Here's how the part is built. I have some questions about the finished solid (model axes, mm). Face numbers are marked on the shaded views. A direction names the side the tool comes from. Give positions to 0.01 mm unless a question says otherwise; leave off trailing zeros. Loops run counter-clockwise (first coordinate to the right, second up) from the corner with the lowest first, then second, coordinate; pieces in that order, holes last. Notation, with made-up numbers: M 70.25,50.25 L 80.25,50.25 A21 cw 80.25,86.25 Z; hole C 45,47.25 d4. An arc over 180 degrees is marked long. Answer as CSV lines item,"result". Start each with the question number.
Item 1: I want a section at A-A on x = -15.5. List the corners of the cut face in (y, z) for me.
Item 2: If I drill on line 1 along X through (y, z) = (-2.5, 1); line 2 along Y through (x, z) = (-15.5, -3.25); line 3 along Y through (x, z) = (-6.5, 0.75), over which ranges is the centre line in solid material (lowest first)? Write a range as from..to.
Item 3: I want a section at C-C on y = 4.75. List the corners of the cut face in (x, z) for me, plus the area to 3 significant figures.
Item 4: If we mould it in two halves opening along Y, with no side actions, what happens to the marked faces 3, 4 and 5? For each: released by +Y, released by -Y, zero draft, split by the parting line, or undercut.
Item 5: I want a section at B-B on x = 10. List the corners of the cut face in (y, z) for me, plus the area to 3 significant figures.
Item 6: I want a section at D-D on z = -4. Give the number of separate pieces and of enclosed holes in the cut face, plus the area to 3 significant figures.
Item 7: For the marked faces 1 and 2, which set-ups out of +Z, -Z, +X, -X, +Y, -Y let a thin tool reach every point of the face, with its end or its side?
Item 8: Will these pins go through, and if not, where does the flat tip stop? P1, Ø0.6, axis at x = 4.5, y = -4.5, coming from the -Z side; P2, Ø1, axis at x = 6, z = -5, coming from the +Y side; P3, Ø5, axis at x = 5, y = 9.5, coming from the +Z side.
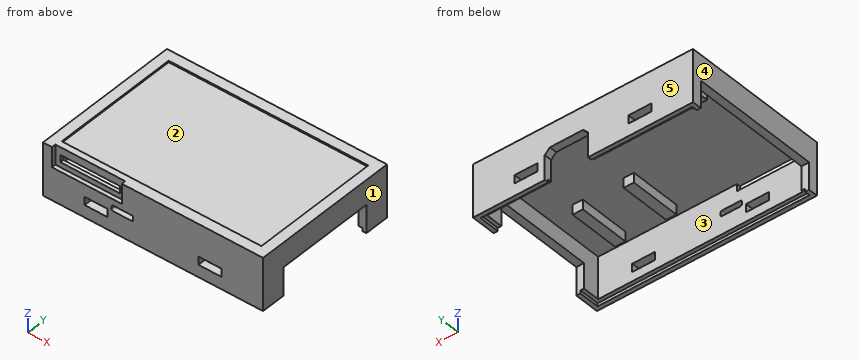
Autodesk Inventor part; units mm, degrees
ref_plane "EbeneAuflage" through (-20, -13, 0) normal (0, 0, 1) x (1, 0, 0)
ref_plane "YZ Plane" through (0, 0, 0) normal (1, 0, 0) x (0, 1, 0)
ref_plane "XZ Plane" through (0, 0, 0) normal (0, 1, 0) x (-1, 0, 0)
ref_plane "EbeneBoden" through (-11.5031, -4.6031, 1.9) normal (0, 0, 1) x (1, 0, 0)
ref_plane "EbeneWändeEnde" through (17.7, 4.9, -6.9) normal (0, 0, -1) x (-1, 0, 0)
sketch "SkizzeBoden" plane through (-11.5031, -4.6031, 1.9) normal (0, 0, 1) x (1, 0, 0)
  line L0 (-7.1969, 7.4031) -> (6.8031, 7.4031)
  line L1 (6.8031, 7.4031) -> (6.8031, -7.7969)
  line L2 (6.8031, -7.7969) -> (4.3031, -7.7969)
  line L3 (4.3031, -7.7969) -> (4.3031, -6.7969)
  line L4 (4.3031, -6.7969) -> (-7.1969, -6.7969)
  line L5 (-7.1969, -6.7969) -> (-7.1969, 7.4031)
  line L6 (31.5031, 17.6031) -> (-8.4969, 17.6031)
  line L7 (-8.4969, 17.6031) -> (-8.4969, -8.3969)
  line L8 (-8.4969, -8.3969) -> (31.5031, -8.3969)
  line L9 (31.5031, -8.3969) -> (31.5031, 17.6031)
  line L10 (-18.6669, 4.6031) -> (41.6731, 4.6031)
  line L11 (11.5031, -15.7669) -> (11.5031, 24.9731)
  line L12 (-10.0469, 19.1531) -> (33.0531, 19.1531)
  line L13 (33.0531, 19.1531) -> (33.0531, -9.9469)
  line L14 (33.0531, -9.9469) -> (-10.0469, -9.9469)
  line L15 (-10.0469, -9.9469) -> (-10.0469, 19.1531)
  point P0 (11.5031, 4.6031)
  dimension "d0" = 1.55
extrude "Boden" add sketch "SkizzeBoden" along normal blind 1.5
sketch "SkizzeWände" plane through (-11.5031, -4.6031, 1.9) normal (0, 0, -1) x (-1, 0, 0)
  line L0 (10.0469, 19.1531) -> (-33.0531, 19.1531)
  line L1 (-33.0531, 19.1531) -> (-33.0531, -9.9469)
  line L2 (-33.0531, -9.9469) -> (10.0469, -9.9469)
  line L3 (10.0469, -9.9469) -> (10.0469, 19.1531)
  line L4 (-31.5531, 17.6531) -> (8.5469, 17.6531)
  line L5 (8.5469, 17.6531) -> (8.5469, -8.4469)
  line L6 (8.5469, -8.4469) -> (-31.5531, -8.4469)
  line L7 (-31.5531, -8.4469) -> (-31.5531, 17.6531)
  point P0 (-11.5031, 4.6031)
  dimension "d3" = 1.5
extrude "Wände" add sketch "SkizzeWände" along normal up to surface (8.8 mm away)
sketch "SkizzeAuflage" plane through (-11.5031, -4.6031, 1.9) normal (0, 0, -1) x (-1, 0, 0)
  line L0 (8.5469, -8.4469) -> (8.5469, 17.6531)
  line L1 (-31.5531, -8.4469) -> (8.5469, -8.4469)
  line L2 (-31.5531, 17.6531) -> (-31.5531, -8.4469)
  line L3 (8.5469, 17.6531) -> (-31.5531, 17.6531)
  line L4 (10.0469, 19.1531) -> (10.0469, -9.9469)
  line L5 (-33.0531, 19.1531) -> (10.0469, 19.1531)
  line L6 (-33.0531, -9.9469) -> (-33.0531, 19.1531)
  line L7 (10.0469, -9.9469) -> (-33.0531, -9.9469)
  line L8 (-26.5531, 3.5531) -> (-24.5531, 3.5531)
  line L9 (-24.5531, 3.5531) -> (-24.5531, -6.4469)
  line L10 (-24.5531, -6.4469) -> (-26.5531, -6.4469)
  line L11 (-26.5531, -6.4469) -> (-26.5531, 3.5531)
  line L12 (-16.5531, 3.5531) -> (-14.5531, 3.5531)
  line L13 (-14.5531, 3.5531) -> (-14.5531, -6.4469)
  line L14 (-14.5531, -6.4469) -> (-16.5531, -6.4469)
  line L15 (-16.5531, -6.4469) -> (-16.5531, 3.5531)
  line L16 (6.5469, 13.6531) -> (-13.4531, 13.6531)
  line L17 (-13.4531, 13.6531) -> (-13.4531, 11.6531)
  line L18 (-13.4531, 11.6531) -> (6.5469, 11.6531)
  line L19 (6.5469, 11.6531) -> (6.5469, 13.6531)
  point P0 (-11.5031, 4.6031)
  dimension "d6" = 5
  dimension "d7" = 2
  dimension "d8" = 8
  dimension "d9" = 2
  dimension "d10" = 10
  dimension "d11" = 20
  dimension "d12" = 2
  dimension "d13" = 4
  dimension "d14" = 2
ref_plane "EbeneAuflage" through (-20, -13, 0) normal (0, 0, 1) x (1, 0, 0)
extrude "Auflage" add sketch "SkizzeAuflage" along normal up to surface (1.9 mm away) contours L8 L9 L10 L11 | L12 L13 L14 L15 | L19 L18 L17 L16
sketch "SkizzeSD" plane through (-21.55, -14.55, 3.4) normal (0, -1, 0) x (1, 0, 0)
  line L0 (43.1, 0) -> (43.1, -10.3)
  line L1 (3.05, -2.6) -> (14.15, -2.6)
  line L2 (14.15, -2.6) -> (14.15, -1.6)
  line L3 (14.15, -1.6) -> (3.05, -1.6)
  line L4 (3.05, -1.6) -> (3.05, -2.6)
  line L5 (41.6, -1.5) -> (1.5, -1.5)
  line L6 (14.45, -1.5) -> (2.75, -1.5)
  line L7 (2.75, -1.5) -> (2.75, -2.9)
  line L8 (2.75, -2.9) -> (14.45, -2.9)
  line L9 (14.45, -2.9) -> (14.45, -1.5)
  line L10 (8.6, -4) -> (8.6, -0.8838) construction
  point P0 (21.55, -3.4)
  point P1 (8.6, -2.6)
  dimension "d17" = 0.3
  dimension "d18" = 0.3
extrude "SD" cut sketch "SkizzeSD" against normal up to surface (1.5 mm away) contours L4 L3 L2 L1 | L9 L8 L7 L5
sketch "Skizze7" plane through (-21.55, -14.55, 3.4) normal (0, -1, 0) x (1, 0, 0)
  line L0 (14.45, -1.5) -> (14.45, -2.9)
  line L1 (14.45, -2.9) -> (2.75, -2.9)
  line L2 (0, 0) -> (43.1, 0)
  line L3 (15.45, -3.9) -> (1.75, -3.9)
  line L4 (1.75, -3.9) -> (1.75, 0)
  line L5 (1.75, 0) -> (15.45, 0)
  line L6 (15.45, 0) -> (15.45, -3.9)
  line L7 (8.6, -3.6567) -> (8.6, -1) construction
  point P0 (21.55, -3.4)
  point P1 (8.6, -2.9)
  dimension "d21" = 1
  dimension "d22" = 1
extrude "SDHilfe" cut sketch "Skizze7" against normal blind 0.8
sketch "SkizzeLED" plane through (-21.55, -14.55, -6.9) normal (0, -1, 0) x (1, 0, 0)
  line L0 (16.55, 5.2) -> (17.55, 5.2)
  line L1 (16.55, 5.2) -> (16.55, 4.1)
  line L2 (17.55, 4.1) -> (16.55, 4.1)
  line L3 (17.55, 5.2) -> (17.55, 4.1)
  line L4 (15.05, 5.2) -> (16.05, 5.2)
  line L5 (15.05, 5.2) -> (15.05, 4.1)
  line L6 (16.05, 4.1) -> (15.05, 4.1)
  line L7 (16.05, 5.2) -> (16.05, 4.1)
  line L8 (13.55, 5.2) -> (14.55, 5.2)
  line L9 (13.55, 5.2) -> (13.55, 4.1)
  line L10 (14.55, 4.1) -> (13.55, 4.1)
  line L11 (14.55, 5.2) -> (14.55, 4.1)
  line L12 (15.55, 3.5363) -> (15.55, 5.4531) construction
  line L13 (17.65, 4.1) -> (13.45, 4.1)
  line L14 (13.45, 4.1) -> (13.45, 5.2)
  line L15 (13.45, 5.2) -> (17.65, 5.2)
  line L16 (17.65, 5.2) -> (17.65, 4.1)
  line L17 (41.55, 5.2) -> (1.55, 5.2)
  point P0 (21.55, 6.9)
  point P1 (15.55, 4.1)
  dimension "d25" = 0.1
extrude "LED" cut sketch "SkizzeLED" against normal up to surface (1.5 mm away)
fillet "RundungLED" radius 0.3 4 edges at (-8.1, -13.8, -2.8) (-3.9, -13.8, -2.8) (-8.1, -13.8, -1.7) (-3.9, -13.8, -1.7)
sketch "SkizzeUSB" plane through (-21.55, 14.55, 3.4) normal (0, 1, 0) x (1, 0, 0)
  line L0 (43.1, 10.3) -> (0, 10.3)
  ellipse E0 centre (28.223, 7.641) end of major axis (28.5465, 8.1263) minor radius 0.5 (28.75, 7.72) -> (28.2975, 8.2) ccw
  line L1 (28.2975, 8.2) -> (21.3025, 8.2)
  ellipse E1 centre (21.377, 7.641) end of major axis (21.0535, 8.1263) minor radius 0.5 (21.3025, 8.2) -> (20.85, 7.72) ccw
  line L2 (20.85, 7.72) -> (20.85, 5.9068)
  line L3 (21.8935, 4.8) -> (20.85, 5.9068)
  line L4 (21.8935, 4.8) -> (27.7065, 4.8)
  line L5 (28.75, 5.9068) -> (27.7065, 4.8)
  line L6 (28.75, 5.9068) -> (28.75, 7.72)
  ellipse E2 centre (28.223, 7.641) end of major axis (28.5465, 8.1263) minor radius 0.5 (28.75, 7.72) -> (28.2975, 8.2) ccw
  line L7 (28.2975, 8.2) -> (21.3025, 8.2)
  ellipse E3 centre (21.377, 7.641) end of major axis (21.0535, 8.1263) minor radius 0.5 (21.3025, 8.2) -> (20.85, 7.72) ccw
  line L8 (20.85, 7.72) -> (20.85, 5.9068)
  line L9 (21.8935, 4.8) -> (20.85, 5.9068)
  line L10 (21.8935, 4.8) -> (27.7065, 4.8)
  line L11 (28.75, 5.9068) -> (27.7065, 4.8)
  line L12 (28.75, 5.9068) -> (28.75, 7.72)
  line L13 (20.55, 10.3) -> (29.05, 10.3)
  line L14 (29.05, 10.3) -> (29.05, 4.5)
  line L15 (29.05, 4.5) -> (20.55, 4.5)
  line L16 (20.55, 4.5) -> (20.55, 10.3)
  line L17 (24.8, 8.6856) -> (24.8, 4.4469) construction
  point P0 (21.55, 3.4)
  point P1 (24.8, 8.2)
  dimension "d29" = 0.3
  dimension "d30" = 0.3
extrude "USB" cut sketch "SkizzeUSB" against normal up to surface (1.5 mm away) contours L14 L15 L16 L0 | L6 L5 L4 L3 L2 E1 L1 E0
chamfer "FaseUSB" distance 1 angle 45 2 edges at (7.5, 13.8, -1.1) (-1, 13.8, -1.1)
sketch "Skizze10" plane through (-21.55, -14.55, 3.4) normal (-1, 0, 0) x (0, 0, 1)
  line L0 (-10.3, 29.1) -> (-10.3, 0)
  line L1 (-5.1, 26.95) -> (-5.1, 11.95)
  line L2 (-5.1, 26.95) -> (-8.8, 26.95)
  line L3 (-8.8, 11.95) -> (-8.8, 26.95)
  line L4 (-5.1, 11.95) -> (-8.8, 11.95)
  line L5 (-5.1, 11.15) -> (-5.1, 2.15)
  line L6 (-5.1, 11.15) -> (-8.8, 11.15)
  line L7 (-8.8, 2.15) -> (-8.8, 11.15)
  line L8 (-5.1, 2.15) -> (-8.8, 2.15)
  line L9 (-5, 1.85) -> (-10.3, 1.85)
  line L10 (-10.3, 1.85) -> (-10.3, 27.25)
  line L11 (-10.3, 27.25) -> (-5, 27.25)
  line L12 (-5, 27.25) -> (-5, 1.85)
  line L13 (0, 29.1) -> (0, 0)
  line L14 (-10.3, 29.1) -> (0, 29.1)
  line L15 (3, 14.55) -> (-13.529, 14.55) construction
  line L16 (-8.4, 2.55) -> (-8.4, 10.75)
  line L17 (-8.4, 10.75) -> (-5.5, 10.75)
  line L18 (-5.5, 10.75) -> (-5.5, 2.55)
  line L19 (-5.5, 2.55) -> (-8.4, 2.55)
  line L20 (-8.4, 12.35) -> (-8.4, 26.55)
  line L21 (-8.4, 26.55) -> (-5.5, 26.55)
  line L22 (-5.5, 26.55) -> (-5.5, 12.35)
  line L23 (-5.5, 12.35) -> (-8.4, 12.35)
  point P0 (-3.4, 14.55)
  point P1 (0, 14.55)
  dimension "d36" = 0.3
  dimension "d38" = 0.1
extrude "JSTFC" cut sketch "Skizze10" against normal up to surface (1.5 mm away) contours L11 L12 L9 L0 | L1 L4 L3 L2 | L5 L8 L7 L6 | L16 L17 L18 L19 | L20 L21 L22 L23
sketch "Skizze11" plane through (21.55, -14.55, 3.4) normal (1, 0, 0) x (0, 0, -1)
  line L0 (10.3, 0) -> (10.3, 29.1)
  line L1 (13.0125, 14.55) -> (-3.6442, 14.55) construction
  line L2 (5.1, 14.95) -> (5.1, 23.95)
  line L3 (5.1, 14.95) -> (8.8, 14.95)
  line L4 (8.8, 23.95) -> (8.8, 14.95)
  line L5 (5.1, 23.95) -> (8.8, 23.95)
  line L6 (5.1, 5.15) -> (5.1, 14.15)
  line L7 (5.1, 5.15) -> (8.8, 5.15)
  line L8 (8.8, 14.15) -> (8.8, 5.15)
  line L9 (5.1, 14.15) -> (8.8, 14.15)
  line L10 (10.3, 24.25) -> (4.8, 24.25)
  line L11 (4.8, 24.25) -> (4.8, 4.85)
  line L12 (4.8, 4.85) -> (10.3, 4.85)
  line L13 (10.3, 4.85) -> (10.3, 24.25)
  point P0 (3.4, 14.55)
  point P1 (10.3, 14.55)
  dimension "d41" = 0.3
  dimension "d42" = 0.3
extrude "JSTOSD" cut sketch "Skizze11" against normal up to surface (1.5 mm away) contours L12 L11 L10 L0 | L2 L5 L4 L3 | L6 L9 L8 L7
sketch "Skizze12" plane through (21.55, -14.55, -6.9) normal (0, 0, -1) x (-1, 0, 0)
  line L0 (0, 0) -> (0, 4.85)
  line L1 (43.1, 0) -> (0, 0)
  line L2 (21.55, -5.82) -> (21.55, 34.92)
  line L3 (51.72, 14.55) -> (-8.62, 14.55)
  line L4 (0.8, 28.3) -> (42.3, 28.3)
  line L5 (42.3, 28.3) -> (42.3, 0.8)
  line L6 (42.3, 0.8) -> (0.8, 0.8)
  line L7 (0.8, 0.8) -> (0.8, 28.3)
  point P0 (21.55, 14.55)
  dimension "d45" = 0.8
  dimension "d46" = 0.8
extrude "Lippe" cut sketch "Skizze12" against normal blind 0.6
sketch "SkizzeSchnapper" plane through (-21.55, -14.55, -6.9) normal (0, -1, 0) x (1, 0, 0)
  line L0 (36.15, 5.2) -> (41.55, 5.2)
  line L1 (36.15, 5.2) -> (36.15, 1.5)
  line L2 (42.35, 1.5) -> (36.15, 1.5)
  line L3 (42.35, 5.2) -> (42.35, 1.5)
  line L4 (41.55, 5.2) -> (42.35, 5.2)
  line L5 (0.75, 5.2) -> (1.55, 5.2)
  line L6 (0.75, 5.2) -> (0.75, 1.5)
  line L7 (6.95, 1.5) -> (0.75, 1.5)
  line L8 (6.95, 5.2) -> (6.95, 1.5)
  line L9 (1.55, 5.2) -> (6.95, 5.2)
  ellipse E0 centre (28.223, 2.659) end of major axis (28.5465, 2.1737) minor radius 0.5 (28.2975, 2.1) -> (28.75, 2.58) ccw
  line L10 (28.2975, 2.1) -> (21.3025, 2.1)
  ellipse E1 centre (21.377, 2.659) end of major axis (21.0535, 2.1737) minor radius 0.5 (20.85, 2.58) -> (21.3025, 2.1) ccw
  line L11 (20.85, 2.58) -> (20.85, 4.3932)
  line L12 (21.8935, 5.5) -> (20.85, 4.3932)
  line L13 (21.8935, 5.5) -> (27.7065, 5.5)
  line L14 (28.75, 4.3932) -> (27.7065, 5.5)
  line L15 (28.75, 4.3932) -> (28.75, 2.58)
  line L16 (34.95, 2.4) -> (30.45, 2.4)
  line L17 (30.45, 2.4) -> (30.45, 4)
  line L18 (30.45, 4) -> (34.95, 4)
  line L19 (34.95, 4) -> (34.95, 2.4)
  line L20 (21.55, -2.06) -> (21.55, 12.36)
  line L21 (1.5, 0.6) -> (0.8, 0.6)
  line L22 (41.6, 0.6) -> (1.5, 0.6)
  line L23 (42.3, 0.6) -> (41.6, 0.6)
  line L24 (0.8, 0.6) -> (42.3, 0.6)
  line L25 (41.55, 5.2) -> (1.55, 5.2)
  line L26 (8.15, 2.4) -> (12.65, 2.4)
  line L27 (12.65, 2.4) -> (12.65, 4)
  line L28 (12.65, 4) -> (8.15, 4)
  line L29 (8.15, 4) -> (8.15, 2.4)
  point P0 (21.55, 6.9)
  dimension "d49" = 4.5
  dimension "d50" = 1.8
  dimension "d51" = 1.2
  dimension "d52" = 1.6
  dimension "d53" = 1.2
extrude "Schnapper" cut sketch "SkizzeSchnapper" against normal up to surface (29.1 mm away) contours L16 L17 L18 L19 | L29 L28 L27 L26
sketch "SkizzeAufkleber" plane through (-11.5031, -4.6031, 3.4) normal (0, 0, 1) x (1, 0, 0)
  line L0 (33.0531, 19.1531) -> (-10.0469, 19.1531)
  line L1 (-10.0469, 19.1531) -> (-10.0469, -9.9469)
  line L2 (11.5031, -15.7669) -> (11.5031, 24.9731)
  line L3 (-18.6669, 4.6031) -> (41.6731, 4.6031)
  line L4 (-8.0469, 17.1531) -> (31.0531, 17.1531)
  line L5 (31.0531, 17.1531) -> (31.0531, -7.9469)
  line L6 (31.0531, -7.9469) -> (-8.0469, -7.9469)
  line L7 (-8.0469, -7.9469) -> (-8.0469, 17.1531)
  point P0 (11.5031, 4.6031)
  dimension "d56" = 2
  dimension "d57" = 2
extrude "Aufkleber" cut sketch "SkizzeAufkleber" against normal blind 0.3 contours L4 L5 L3 L2 | L2 L3 L7 L4 | L3 L5 L6 L2 | L2 L6 L7 L3
properties part number "Boden"
Result:
1,outline,"M -14.55,-6.9 L -13.75,-6.9 L -13.75,-6.3 L -13.05,-6.3 L -13.05,0.5 L -13.75,0.5 L -13.75,-0.5 L -14.55,-0.5 Z; M -13.75,1.9 L 7.05,1.9 L 7.05,0 L 9.05,0 L 9.05,1.9 L 13.05,1.9 L 13.05,-6.3 L 13.75,-6.3 L 13.75,-6.9 L 14.55,-6.9 L 14.55,3.4 L 12.55,3.4 L 12.55,3.1 L -12.55,3.1 L -12.55,3.4 L -13.75,3.4 Z"
2,line 1,"-21.55..-20.05, 3.05..5.05, 13.05..15.05, 20.05..21.55"
2,line 2,"-14.55..-13.05, 13.05..14.55"
2,line 3,"-13.75..-13.05, 7.05..9.05, 13.05..14.55"
3,outline,"M -21.55,-1.6 L -20.05,-1.6 L -20.05,1.9 L 20.05,1.9 L 20.05,-1.4 L 21.55,-1.4 L 21.55,3.4 L 19.55,3.4 L 19.55,3.1 L -19.55,3.1 L -19.55,3.4 L -21.55,3.4 Z"
3,area,"63.1 mm^2"
4,face 3,"undercut"
4,face 4,"zero draft"
4,face 5,"released by +Y"
5,outline,"M -14.55,-6.9 L -13.75,-6.9 L -13.75,-6.3 L -13.05,-6.3 L -13.05,-4.5 L -14.55,-4.5 Z; M -14.55,-2.9 L -13.05,-2.9 L -13.05,1.9 L 13.05,1.9 L 13.05,-2.9 L 14.55,-2.9 L 14.55,3.4 L 12.55,3.4 L 12.55,3.1 L -12.55,3.1 L -12.55,3.4 L -14.55,3.4 Z; M 13.05,-6.3 L 13.75,-6.3 L 13.75,-6.9 L 14.55,-6.9 L 14.55,-4.5 L 13.05,-4.5 Z"
5,area,"56.9 mm^2"
6,separate pieces,"7"
6,enclosed holes,"0"
6,area,"101 mm^2"
7,face 1,"+Z, -Z, +X, +Y, -Y"
7,face 2,"+Z"
8,P1,"z = 0"
8,P2,"y = -13.05"
8,P3,"z = 3.1"
